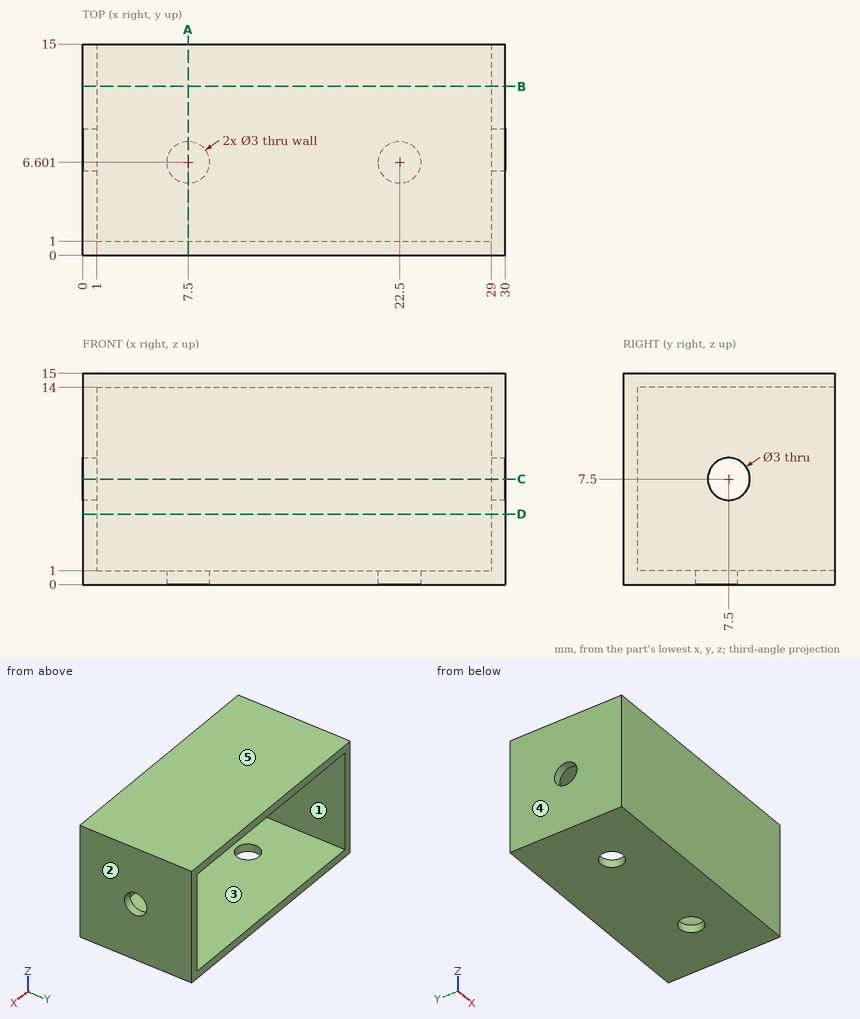
Could you check a few things on this drawing? It's one solid part, dimensions in mm from its lowest x, y, z. A direction names the side the tool comes from. Coordinates: 2 decimals unless noted, no trailing zeros. Order: outer loops, then holes, each group sorted by start corner. A loop starts at its lowest first (then second) coordinate and runs counter-clockwise, first axis right, second up. Notation, with made-up numbers: (56, 57) -> (91, 57) arc R30 ccw to (91, 85) -> close; hole circle Ø7 at (65, 27). An arc over 180 degrees is marked (long way). Answer in a Markdown table with one row per item.
(1) On a 3-axis mill with a long thin cutter (end or side, diameter ignored), from which of +Z, -Z, +X, -X, +Y, -Y can I reach the whole of each face in a straight line? I mean the marked faces 1 and 2. Say none if no direction works.
Answer key:
| item | result |
|---|---|
| face 1 | +Y |
| face 2 | +Z, -Z, +X, +Y, -Y |
(2) Please list where these lines run through material, in increasing order: probe 1 along X at (y, z) = (5, 2.25); probe 2 along Y at (x, z) = (0.3, 7.5); probe 3 along Y at (x, z) = (22.5, 0.45).
Answer key:
| item | result |
|---|---|
| probe 1 | 0 to 1, 29 to 30 |
| probe 2 | 0 to 6, 9 to 15 |
| probe 3 | 0 to 5.1, 8.1 to 15 |
(3) I want a section at A-A on x = 7.5. List the corners of the cut face in (y, z) for me, then the cut area to 3 significant figures.
Answer key:
| item | result |
|---|---|
| outline | (0, 0) -> (5.1, 0) -> (5.1, 1) -> (1, 1) -> (1, 14) -> (15, 14) -> (15, 15) -> (0, 15) -> close; (8.1, 0) -> (15, 0) -> (15, 1) -> (8.1, 1) -> close |
| area | 40.0 mm^2 |
(4) I want a section at D-D on z = 5. List the corners of the cut face in (x, y) for me.
Answer key:
| item | result |
|---|---|
| outline | (0, 0) -> (30, 0) -> (30, 15) -> (29, 15) -> (29, 1) -> (1, 1) -> (1, 15) -> (0, 15) -> close |
(5) I want a section at C-C on z = 7.5. List the corners of the cut face in (x, y) for me.
Answer key:
| item | result |
|---|---|
| outline | (0, 0) -> (30, 0) -> (30, 6) -> (29, 6) -> (29, 1) -> (1, 1) -> (1, 6) -> (0, 6) -> close; (0, 9) -> (1, 9) -> (1, 15) -> (0, 15) -> close; (29, 9) -> (30, 9) -> (30, 15) -> (29, 15) -> close |
(6) Will these pins go through, and if not, where does the flat tip stop? pin 1 Ø1.5 at (x, y) = (6, 7.5) entering from -Z; pin 2 Ø2 at (x, z) = (16, 6.5) entering from +Y; pin 3 Ø1.8 at (y, z) = (7.5, 7.5) entering from -X; pin 4 Ø1.8 at (x, y) = (7.5, 6.6) entering from -Z.
Answer key:
| item | result |
|---|---|
| pin 1 | z = 0 |
| pin 2 | y = 1 |
| pin 3 | through |
| pin 4 | z = 14 |
(7) I want a section at B-B on y = 12. List the corners of the cut face in (x, z) for me.
Answer key:
| item | result |
|---|---|
| outline | (0, 0) -> (30, 0) -> (30, 15) -> (0, 15) -> close; hole (1, 1) -> (29, 1) -> (29, 14) -> (1, 14) -> close |
(8) Thinking about a two-plate mould opening in X: for the marked faces 3, 4 and 5, which applies, +X half, -X half, draft (parallel to the pull), parting line (faces both ways), or undercut?
Answer key:
| item | result |
|---|---|
| face 3 | undercut |
| face 4 | -X half |
| face 5 | draft |
